from build123d import *

# Parameters (mm, degrees)
F0_W     = 80
F0_H     = 12
F1_DEPTH = 12
F3_R     = 5
F4_DEPTH = 25
F2_R     = 5
F5_DEPTH = 25
F6_R     = 1.6
F6_R_2   = 1.8
F7_DEPTH = 25


with BuildPart() as f1:
    # F0 (on Front) → F1 (new body)
    with BuildSketch(Plane.XZ):
        with Locations((40, 6)):
            Rectangle(F0_W, F0_H)
    extrude(amount=F1_DEPTH)

    # F3 (on face) → F4 (cut)
    with BuildSketch(Plane.XY.offset(12)):
        with Locations((44.75, -6)):
            Circle(F3_R)
    extrude(amount=-F4_DEPTH, mode=Mode.SUBTRACT)

    # F2 (on face) → F5 (cut)
    with BuildSketch(Plane.XY.offset(12)):
        with Locations((35.25, -6)):
            Circle(F2_R)
    extrude(amount=-F5_DEPTH, mode=Mode.SUBTRACT)

    # F6 (on face) → F7 (cut)
    with BuildSketch(Plane(origin=(0, 0, 0), x_dir=(-1, 0, 0), z_dir=(0, 1, 0))):
        with Locations((-5, 6)):
            Circle(F6_R)
        with Locations((-20, 6)):
            Circle(F6_R)
        with Locations((-75, 6)):
            Circle(F6_R_2)
        with Locations((-60, 6)):
            Circle(F6_R_2)
    extrude(amount=-F7_DEPTH, mode=Mode.SUBTRACT)


solid = f1.part
Input: part model. Units: mm. Frame: model coordinates. Give positions to 0.01 mm unless a question says otherwise; leave off trailing zeros. Write each loop counter-clockwise with the first axis right and the second up, starting at its lowest first coordinate (ties: lowest second). Pieces come first, ordered by that corner, then holes. Notation, with made-up numbers: (10.25, 21.5) -> (18.25, 21.5) arc R18 ccw to (18.25, 36.5) -> close; hole circle Ø8 at (3, -30.75). An arc over 180 degrees is marked (long way). Use one line per item in the form item = value. Start each with the question number.
1) Ray query, probe 1 along Y at (x, z) = (45, 7.75); probe 2 along X at (y, z) = (-6, 8.5); probe 3 along Z at (x, y) = (5, -6.25). Return the intervals inside material, ascending. Write a range as from..to.
2) Section query D-D on x = 60. Return the cut outline in (y, z).
3) Draft query along Z for faces 1 (the cylindrical face through (21.27, -5.92, 5.03)), 2 (the flat face through (39, -2, 12)), 3 (the flat face through (39, -2, 0)), 4 (the flat face through (39, 0, 6)). Return one class per face: pulls with the +Z half, pulls with the -Z half, needs draft (parallel to the pull), parting line crosses it, or undercut.
4) Section query C-C on y = -6. Return the cut outline in (x, z), then the cut area to 3 significant figures.
5) Pin query (flat end, axial travel): pin 1 (3 mm diameter, centred on x = 60, z = 6, fed in from +Y). Return the tip coordinate at first contact, or that it passes through.
6) Section query B-B on x = 20. Return the cut outline in (y, z), then the cut area to 3 significant figures.
7) Section query A-A on y = -3. Return the cut outline in (x, z), then the cut area to 3 significant figures.
Outcome:
q1.probe_1 = -12..-10.99, -1.01..0
q1.probe_2 = 0..30.25, 49.75..80
q1.probe_3 = 0..4.4, 7.6..12
q2.outline = (-12, 0) -> (0, 0) -> (0, 4.2) -> (-12, 4.2) -> close; (-12, 7.8) -> (0, 7.8) -> (0, 12) -> (-12, 12) -> close
q3.face_1 = undercut
q3.face_2 = pulls with the +Z half
q3.face_3 = pulls with the -Z half
q3.face_4 = needs draft
q4.outline = (0, 0) -> (30.25, 0) -> (30.25, 12) -> (0, 12) -> close; (49.75, 0) -> (80, 0) -> (80, 12) -> (49.75, 12) -> close; hole circle Ø3.2 at (5, 6); hole circle Ø3.2 at (20, 6); hole circle Ø3.6 at (60, 6); hole circle Ø3.6 at (75, 6)
q4.area = 690 mm^2
q5.pin_1 = through
q6.outline = (-12, 0) -> (0, 0) -> (0, 4.4) -> (-12, 4.4) -> close; (-12, 7.6) -> (0, 7.6) -> (0, 12) -> (-12, 12) -> close
q6.area = 106 mm^2
q7.outline = (0, 0) -> (31.25, 0) -> (31.25, 12) -> (0, 12) -> close; (39.25, 0) -> (40.75, 0) -> (40.75, 12) -> (39.25, 12) -> close; (48.75, 0) -> (80, 0) -> (80, 12) -> (48.75, 12) -> close; hole circle Ø3.2 at (5, 6); hole circle Ø3.2 at (20, 6); hole circle Ø3.6 at (60, 6); hole circle Ø3.6 at (75, 6)
q7.area = 732 mm^2
